Source: CAD feature listing. Evaluate the final solid. Frame: model axes, mm. Face numbers are marked on the shaded views. A direction names the side the tool comes from. Give positions to 0.01 mm unless a question says otherwise; leave off trailing zeros. Order: outer loops, then holes, each group sorted by start corner. A loop starts at its lowest first (then second) coordinate and runs counter-clockwise, first axis right, second up. Notation, with made-up numbers: M 83.5,-17 L 115.5,-17 A17 cw 115.5,14 Z; hole C -3,59 d5. An arc over 180 degrees is marked long. Answer in a Markdown table with one row per item. Add a question column.
(1) Material intervals for line 1 along Y through (x, z) = (3, -8); line 2 along Z through (x, y) = (2, -21.5); line 3 along Z through (x, y) = (-22, -15.5), sorted ascending.
(2) Pin query (flat end, axial travel): P1, Ø10, axis at x = -9, z = -9.5, coming from the +Y side; P2, Ø13, axis at x = -18.5, y = -12, coming from the -Z side; P3, Ø10, axis at x = 1, y = -12, coming from the -Z side; P4, Ø5, axis at x = -1, y = -14.5, coming from the +Z side. Return the tip coordinate at first contact, or that it passes through.
(3) Section query C-C, the plane z = -43. Return loops of the section in (x, y), plus the area to 3 significant figures.
(4) Section query A-A, the plane z = 6.5. Return loops of the section in (x, y), plus the area to 3 significant figures.
(5) Mould query, pull axis X, two halves, no side actions, for the marked faces 1, 2 and 3. Classes: pulls with the +X half, pulls with the -X half, needs draft (parallel to the pull), parting line crosses it, or undercut.
(6) Section query B-B, the plane y = -22. Return loops of the section in (x, z).
(7) Section query D-D, the plane y = -40.5. Return loops of the section in (x, z).
(8) Set-up query: the marked faces 4, 5 and 6. Return all of +Z, -Z, +X, -X, +Y, -Y with unobstructed straight access to the full face (end or side cutting, diameter ignored); none if empty.
from build123d import *

# Parameters (mm, degrees)
SKETCH1_R             = 6
BOSS_EXTRUDE1_DEPTH   = 15
BOSS_EXTRUDE1_2_DEPTH = 15
BOSS_EXTRUDE1_3_DEPTH = 15
BOSS_EXTRUDE2_START   = -3
BOSS_EXTRUDE2_DEPTH   = 13
SKETCH4_R             = 6
BOSS_EXTRUDE3_DEPTH   = 40


with BuildPart() as part:
    # Sketch1 → Boss-Extrude1 (new body)
    with BuildSketch(Plane.XY):
        with Locations((0, -44)):
            Circle(SKETCH1_R)
    extrude(amount=BOSS_EXTRUDE1_DEPTH)



with BuildPart() as body_2:
    # Sketch1 → Boss-Extrude1 2 (new body)
    with BuildSketch(Plane.XY):
        with Locations((19.052558883, -11)):
            Circle(SKETCH1_R)
    extrude(amount=BOSS_EXTRUDE1_2_DEPTH)


with BuildPart() as body_3:
    # Sketch1 → Boss-Extrude1 3 (new body)
    with BuildSketch(Plane.XY):
        with Locations((-19.052558883, -11)):
            Circle(SKETCH1_R)
    extrude(amount=BOSS_EXTRUDE1_3_DEPTH)


with BuildPart() as part_1:
    add(part.part)

    add(body_2.part)  # Boss-Extrude2 merges body 2

    add(body_3.part)  # Boss-Extrude2 merges body 3
    # Sketch2 → Boss-Extrude2 (add)
    with BuildSketch(Plane(origin=(0, 0, 0), x_dir=(-1, 0, 0), z_dir=(0, 0, -1)).offset(BOSS_EXTRUDE2_START)):
        Polygon((-19.052558883, -11), (0, -44), (19.052558883, -11), align=None)
    extrude(amount=BOSS_EXTRUDE2_DEPTH)

    # Sketch4 → Boss-Extrude3 (add)
    with BuildSketch(Plane(origin=(0, 0, -10), x_dir=(-1, 0, 0), z_dir=(0, 0, -1))):
        with Locations((0, -22)):
            Circle(SKETCH4_R)
    extrude(amount=BOSS_EXTRUDE3_DEPTH)


solid = part_1.part
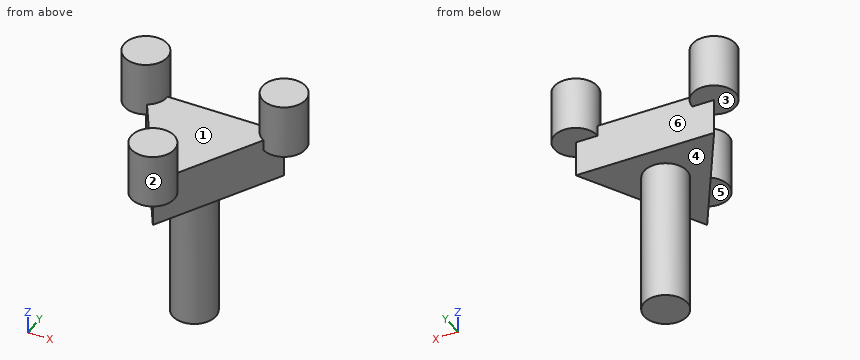
Values follow:
| question | item | result |
|---|---|---|
| 1 | line 1 | y = -38.8 to -11 |
| 1 | line 2 | z = -50 to 3 |
| 1 | line 3 | z = 0 to 15 |
| 2 | P1 | stops at y = -11 |
| 2 | P2 | stops at z = -10 |
| 2 | P3 | stops at z = -50 |
| 2 | P4 | stops at z = 3 |
| 3 | outline | C 0,-22 d12 |
| 3 | area | 113 mm² |
| 4 | outline | C -19.05,-11 d12; C 0,-44 d12; C 19.05,-11 d12 |
| 4 | area | 339 mm² |
| 5 | face 1 | undercut |
| 5 | face 2 | parting line crosses it |
| 5 | face 3 | needs draft |
| 6 | outline | M -12.7,-10 L -6,-10 L -6,-50 L 6,-50 L 6,-10 L 12.7,-10 L 12.7,3 L -12.7,3 Z |
| 7 | outline | M -4.87,0 L -2.02,0 L -2.02,-10 L 2.02,-10 L 2.02,0 L 4.87,0 L 4.87,15 L -4.87,15 Z |
| 8 | face 4 | -Z |
| 8 | face 5 | -Z, -Y |
| 8 | face 6 | -Z, +Y |
